The listing builds one solid part. Answer for the finished solid, in the listing's coordinates (mm). A direction names the side the tool comes from. Round coordinates to 2 decimals unless told otherwise and drop trailing zeros. Order: outer loops, then holes, each group sorted by start corner. A loop starts at its lowest first (then second) coordinate and runs counter-clockwise, first axis right, second up. Notation, with made-up numbers: M -15.5,62 L 32.5,62 A24 cw 32.5,75 Z; hole C 83.5,56.5 d1. An arc over 180 degrees is marked long. Put each result on its own line as item: value. Start each with the question number.
1. Which of the six approach directions +Z, -Z, +X, -X, +Y, -Y give full straight-line access (tool end or side, diameter ignored) to faces 1 (the face through (-14, 23, -76.2)), 2 (the face through (-30.133, 1.326, 5.765))?
2. The mould has two halves that part along X. Classify faces 3 (the face through (28, 12, -6.35)), 4 (the face through (-5.506, -24.796, 15.919)), 5 (the face through (-6.883, 30.995, -40.379)): +X half, -X half, draft (parallel to the pull), parting line (faces both ways), or undercut.
3. Each of these flat-tipped pins is pushed along its axis until it touches: pin 1 Ø10 at (y, z) = (16.5, -12.5) entering from -X; pin 2 Ø2 at (y, z) = (16, -17.5) entering from +X; pin 3 Ø2 at (x, z) = (7.5, 0) entering from -Y. Where does it stop, or does it pass through?
4. Consider line 1 (Y direction, x = -1, z = -34); line 2 (X direction, y = 0.5, z = 8); line 3 (X direction, y = -3.5, z = -1). Determine where each line is inside the solid, lowest interval first.
5. The part is cut by section C-C (z = 2). Give the vertices of the cut face in (x, y) (1 decimal).
6. The part is cut by section D-D (z = -57). Give the vertices of the cut face in (x, y), then the cut area to 3 significant figures.
from build123d import *

# Parameters (mm, degrees)
F0_R     = 30.1625
F1_DEPTH = 6.35
F2_R     = 31.75
F3_DEPTH = 69.85
F4_R     = 30.1625
F5_DEPTH = 12.7
F6_R     = 24.638
F7_DEPTH = 95.251
F8_R     = 25.4
F9_DEPTH = 6.35
F10_SIZE = 0.76199
F11_SIZE = 1.5875
F12_SIZE = 0.8255


# Not quite as in the source:
# - a fillet or chamfer is up to 0.001 mm smaller than in the source, because OpenCascade refuses the exact size


with BuildPart() as f1:
    # F0 (on Top) → F1 (new body, symmetric)
    with BuildSketch(Plane.XY):
        Circle(F0_R)
    extrude(amount=F1_DEPTH, both=True)

    # F2 (on face) → F3 (join)
    with BuildSketch(Plane(origin=(0, 0, -6.35), x_dir=(1, 0, 0), z_dir=(0, 0, -1))):
        Circle(F2_R)
    extrude(amount=F3_DEPTH)

    # F4 (on face) → F5 (join)
    with BuildSketch(Plane.XY.offset(6.35)):
        Circle(F4_R)
    extrude(amount=F5_DEPTH)

    # F6 (on face) → F7 (cut, through all)
    with BuildSketch(Plane.XY.offset(19.05)):
        Circle(F6_R)
    extrude(amount=-F7_DEPTH, mode=Mode.SUBTRACT)

    # F8 (on face) → F9 (cut)
    with BuildSketch(Plane.XY.offset(19.05)):
        Circle(F8_R)
    extrude(amount=-F9_DEPTH, mode=Mode.SUBTRACT)

    # F10 (size 0.762 in the source; OpenCascade refuses exactly that, so slightly less here)
    f10_edges = [f1.edges().sort_by_distance(p)[0] for p in [
        (-24.638, 0, 12.7),
    ]]
    chamfer(f10_edges, length=F10_SIZE)

    # F11
    f11_edges = [f1.edges().sort_by_distance(p)[0] for p in [
        (-24.638, 0, -76.2),
    ]]
    chamfer(f11_edges, length=F11_SIZE)

    # F12
    f12_edges = [f1.edges().sort_by_distance(p)[0] for p in [
        (-31.75, 0, -76.2),
        (-30.1625, 0, 19.05),
    ]]
    chamfer(f12_edges, length=F12_SIZE)


solid = f1.part
Resolved:
1. face 1: -Z, +X, -X, +Y, -Y
1. face 2: +Z
2. face 3: draft
2. face 4: undercut
2. face 5: parting line
3. pin 1: x = -29.59
3. pin 2: x = 27.98
3. pin 3: y = -29.45
4. line 1: -31.73 to -24.62, 24.62 to 31.73
4. line 2: -30.16 to -24.63, 24.63 to 30.16
4. line 3: -29.96 to -24.39, 24.39 to 29.96
5. outline: C 0,0 d60.3; hole C 0,0 d49.3
6. outline: C 0,0 d63.5; hole C 0,0 d49.28
6. area: 1,260 mm2
